Geometry: final body of the model. Coordinates: model frame, mm. Face numbers are marked on the shaded views. A direction names the side the tool comes from. Give positions to 0.01 mm unless a question says otherwise; leave off trailing zeros. Loops run counter-clockwise (first coordinate to the right, second up) from the corner with the lowest first, then second, coordinate; pieces in that order, holes last.
1. Section A-A, the plane y = -24.5. Output: boundary loops of the cut face in (x, z).
2. Material intervals for line 1 along Y through (x, z) = (-9, -24.5); line 2 along X through (y, z) = (-19.5, -17); line 3 along Y through (x, z) = (-5.75, -23), sorted ascending.
3. Section B-B, the plane x = -1.75. Output: boundary loops of the cut face in (y, z), then the cut area to 3 significant figures.
4. Draft query along X for the marked faces 3, 4 and 5. Return one class per face: +X half, -X half, draft (parallel to the pull), parting line (faces both ways), or undercut.
5. First-contact query: P1, Ø0.5, axis at y = -51.5, z = 6, coming from the +X side; P2, Ø2.5, axis at x = 1.5, z = -9.5, coming from the -Y side. Flat tips, straight axial feed; report the tip coordinate or a pass-through.
6. Access query for the marked faces 1 and 2. Directions: +Z, -Z, +X, -X, +Y, -Y. A direction counts if a zero-diameter tool reaches every point of the face in a straight line with its end or side. Return the directions, or none.
from build123d import *

# Parameters (mm, degrees)
EXTRUDE_1_DEPTH = 50


with BuildPart() as part:
    # 草图1 → 凸台-拉伸1 (new, symmetric)
    with BuildSketch(Plane.XY):
        with BuildLine():
            Line((12.49999999, 0), (-12.49999999, 0))
            ThreePointArc((-12.49999999, 0), (-14.267766942, -0.732233047), (-14.999999989, -2.499999998))
            Line((-14.999999989, -2.499999998), (-14.999999989, -50.500000002))
            ThreePointArc((-14.999999989, -50.500000002), (-14.267766942, -52.267766953), (-12.49999999, -53))
            Line((-12.49999999, -53), (-5.399999995, -53))
            ThreePointArc((-5.399999995, -53), (-5.187867961, -52.912132034), (-5.099999996, -52.7))
            Line((-5.099999996, -52.7), (-5.099999996, -52.300000001))
            ThreePointArc((-5.099999996, -52.300000001), (-5.01213203, -52.087867966), (-4.799999996, -52.000000001))
            Line((-4.799999996, -52.000000001), (-4.399999997, -52.000000001))
            ThreePointArc((-4.399999997, -52.000000001), (-4.187867962, -51.912132035), (-4.099999997, -51.700000001))
            Line((-4.099999997, -51.700000001), (-4.099999997, -51.100000001))
            ThreePointArc((-4.099999997, -51.100000001), (-4.187867962, -50.887867967), (-4.399999997, -50.800000002))
            Line((-4.399999997, -50.800000002), (-7.949999994, -50.800000002))
            ThreePointArc((-7.949999994, -50.800000002), (-8.162132028, -50.712132036), (-8.249999994, -50.500000002))
            Line((-8.249999994, -50.500000002), (-8.249999994, -47.929898991))
            ThreePointArc((-8.249999994, -47.929898991), (-8.227163853, -47.815093962), (-8.162132028, -47.717766957))
            Line((-8.162132028, -47.717766957), (-4.332233044, -43.887867973))
            ThreePointArc((-4.332233044, -43.887867973), (-4.234906039, -43.822836147), (-4.12010101, -43.800000007))
            Line((-4.12010101, -43.800000007), (4.12010101, -43.800000007))
            ThreePointArc((4.12010101, -43.800000007), (4.234906039, -43.822836147), (4.332233044, -43.887867973))
            Line((4.332233044, -43.887867973), (8.162132028, -47.717766957))
            ThreePointArc((8.162132028, -47.717766957), (8.227163854, -47.815093961), (8.249999994, -47.929898991))
            Line((8.249999994, -47.929898991), (8.249999994, -50.500000002))
            ThreePointArc((8.249999994, -50.500000002), (8.162132028, -50.712132036), (7.949999994, -50.800000002))
            Line((7.949999994, -50.800000002), (4.399999997, -50.800000002))
            ThreePointArc((4.399999997, -50.800000002), (4.187867963, -50.887867967), (4.099999997, -51.100000001))
            Line((4.099999997, -51.100000001), (4.099999997, -51.700000001))
            ThreePointArc((4.099999997, -51.700000001), (4.187867963, -51.912132035), (4.399999997, -52.000000001))
            Line((4.399999997, -52.000000001), (4.799999996, -52.000000001))
            ThreePointArc((4.799999996, -52.000000001), (5.01213203, -52.087867966), (5.099999996, -52.300000001))
            Line((5.099999996, -52.300000001), (5.099999996, -52.7))
            ThreePointArc((5.099999996, -52.7), (5.187867962, -52.912132034), (5.399999996, -53))
            Line((5.399999996, -53), (12.49999999, -53))
            ThreePointArc((12.49999999, -53), (14.267766942, -52.267766953), (14.999999989, -50.500000002))
            Line((14.999999989, -50.500000002), (14.999999989, -2.499999998))
            ThreePointArc((14.999999989, -2.499999998), (14.267766942, -0.732233047), (12.49999999, 0))
        make_face()
        with BuildLine():
            Line((10.999999989, -2), (-10.999999989, -2))
            ThreePointArc((-10.999999989, -2), (-12.414213551, -2.585786438), (-12.999999989, -4))
            Line((-12.999999989, -4), (-12.999999989, -41.800000007))
            Line((-12.999999989, -41.800000007), (12.999999989, -41.800000007))
            Line((12.999999989, -41.800000007), (12.999999989, -4))
            ThreePointArc((12.999999989, -4), (12.414213551, -2.585786438), (10.999999989, -2))
        make_face(mode=Mode.SUBTRACT)
    extrude(amount=EXTRUDE_1_DEPTH, both=True)


solid = part.part
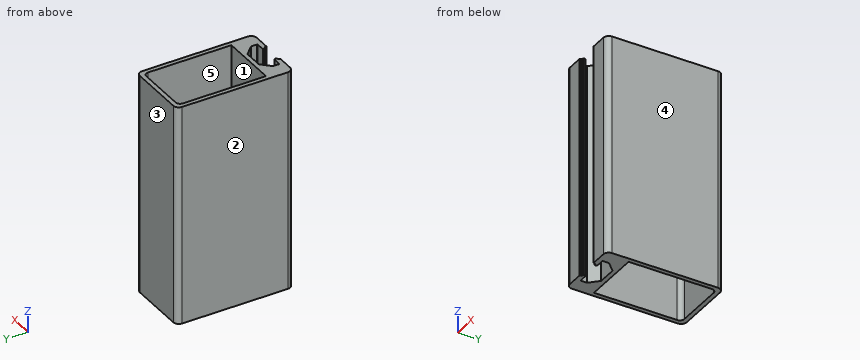
Answers below:
1. outline: (-15, -50) - (-13, -50) - (-13, 50) - (-15, 50) - close; (13, -50) - (15, -50) - (15, 50) - (13, 50) - close
2. line 1: y = -53 to -41.8, -2 to 0
2. line 2: x = -15 to -13, 13 to 15
2. line 3: y = -53 to -50.8, -45.31 to -41.8, -2 to 0
3. outline: (-43.8, -50) - (-41.8, -50) - (-41.8, 50) - (-43.8, 50) - close; (-2, -50) - (0, -50) - (0, 50) - (-2, 50) - close
3. area: 400 mm2
4. face 3: draft
4. face 4: +X half
4. face 5: undercut
5. P1: stops at x = 14.88
5. P2: stops at y = -43.8
6. face 1: +Z, -Z
6. face 2: +Z, -Z, -X, +Y, -Y
